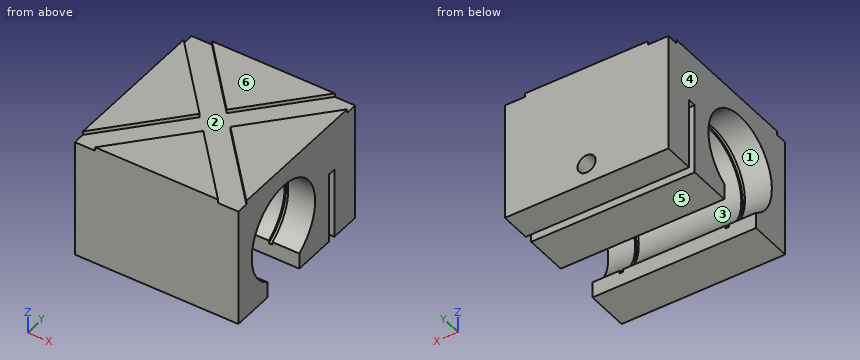
from build123d import *

# Parameters (mm, degrees)
SKETCH3_W               = 67
SKETCH3_H               = 50
BOSS_EXTRUDE1_DEPTH     = 70
CUT_EXTRUDE1_DEPTH      = 110.036691072
CUT_EXTRUDE1_DEPTH_BACK = 1.5
CUT_EXTRUDE3_DEPTH      = 110.036691072
SKETCH8_W               = 29
SKETCH8_H               = 3.3
CUT_EXTRUDE4_DEPTH      = 110.036691072
CUT_EXTRUDE5_REACH      = 111.037
SKETCH4_R               = 3.720223744
SKETCH9_R               = 20
CUT_EXTRUDE6_DEPTH      = 1.5
CUT_EXTRUDE7_START      = -1.5
SKETCH10_R              = 20
CUT_EXTRUDE7_DEPTH      = 1.5


with BuildPart() as part:
    # Sketch3 → Boss-Extrude1 (new body)
    with BuildSketch(Plane(origin=(0, 0, 0), x_dir=(1, 0, 0), z_dir=(0, 1, 0))):
        with Locations((33.5, 25)):
            Rectangle(SKETCH3_W, SKETCH3_H)
    extrude(amount=-BOSS_EXTRUDE1_DEPTH)

    # Sketch5 → Cut-Extrude1 (cut, two sides: drawn at the far end of the back side and taken through both)
    with BuildSketch(Plane.XY.offset(-CUT_EXTRUDE1_DEPTH_BACK)):
        Polygon((27.182851456, -35), (0, -65.2), (0, -70), (8.313843876, -70), (33.5, -42.018317645), (58.686156124, -70), (67, -70), (67, -65.2), (39.817148544, -35), (67, -4.8), (67, 0), (58.686156124, 0), (33.5, -27.981682355), (8.313843876, 0), (0, 0), (0, -4.8), align=None)
    extrude(amount=CUT_EXTRUDE1_DEPTH + CUT_EXTRUDE1_DEPTH_BACK, mode=Mode.SUBTRACT)

    # Sketch6 → Cut-Extrude3 (cut, through all)
    with BuildSketch(Plane(origin=(67, 0, 0), x_dir=(0, 0, -1), z_dir=(1, 0, 0))):
        with BuildLine():
            Line((43.454482672, -33.5), (50, -33.5))
            Line((50, -33.5), (50, -52.5))
            Line((50, -52.5), (43.454482672, -52.5))
            ThreePointArc((43.454482672, -52.5), (8, -43), (43.454482672, -33.5))
        make_face()
    extrude(amount=-CUT_EXTRUDE3_DEPTH, mode=Mode.SUBTRACT)

    # Sketch8 → Cut-Extrude4 (cut, through all)
    with BuildSketch(Plane(origin=(67, 0, 0), x_dir=(0, 0, -1), z_dir=(1, 0, 0))):
        with Locations((35.5, -14.15)):
            Rectangle(SKETCH8_W, SKETCH8_H)
    extrude(amount=-CUT_EXTRUDE4_DEPTH, mode=Mode.SUBTRACT)

    # Sketch4 → Cut-Extrude5 (cut, up to next)
    with BuildSketch(Plane(origin=(0, 0, 0), x_dir=(1, 0, 0), z_dir=(0, 1, 0)), mode=Mode.PRIVATE) as cut_extrude5_sk1:
        with Locations(Location((33.5, 41.7, 0), (0, 0, 270))):
            Circle(SKETCH4_R)
    cut_extrude5_tool1 = extrude(cut_extrude5_sk1.sketch, amount=-CUT_EXTRUDE5_REACH, mode=Mode.PRIVATE) & part.part
    add(cut_extrude5_tool1.solids().sort_by_distance((33.5, 0, -41.7))[0], mode=Mode.SUBTRACT)

    # Sketch9 → Cut-Extrude6 (cut)
    with BuildSketch(Plane(origin=(54.5, 0, 0), x_dir=(0, 0, -1), z_dir=(1, 0, 0))):
        with Locations((27, -43)):
            Circle(SKETCH9_R)
    extrude(amount=CUT_EXTRUDE6_DEPTH, mode=Mode.SUBTRACT)

    # Sketch10 → Cut-Extrude7 (cut)
    with BuildSketch(Plane(origin=(12.5, 0, 0), x_dir=(0, 0, -1), z_dir=(1, 0, 0)).offset(CUT_EXTRUDE7_START)):
        with Locations((27, -43)):
            Circle(SKETCH10_R)
    extrude(amount=CUT_EXTRUDE7_DEPTH, mode=Mode.SUBTRACT)


solid = part.part
The model under review builds one solid part; all positions refer to its coordinate system, in mm. Face numbers are marked on the shaded views. A direction names the side the tool comes from. Round coordinates to 2 decimals unless told otherwise and drop trailing zeros. Loops run counter-clockwise (first coordinate to the right, second up) from the corner with the lowest first, then second, coordinate; pieces in that order, holes last. Notation, with made-up numbers: M 26,70.5 L 36,70.5 A16 cw 36,82.5 Z; hole C 57.25,34 d7. An arc over 180 degrees is marked long. Answer as CSV lines item,"result".
1. We need section C-C (x = 32). Give the boundary of the cut face in (y, z), plus the area to 3 significant figures.
Outcome:
outline,"M -70,-50 L -52.5,-50 L -52.5,-43.45 A19 cw long -33.5,-43.45 L -33.5,-50 L -15.8,-50 L -15.8,-21 L -12.5,-21 L -12.5,-38.3 L 0,-38.3 L 0,0 L -26.32,0 L -26.32,-1.5 L -43.68,-1.5 L -43.68,0 L -70,0 Z; M -12.5,-50 L 0,-50 L 0,-45.1 L -12.5,-45.1 Z"
area,"2,070 mm2"
2. We need section A-A (z = -27). Give the boundary of the cut face in (x, y), plus the area to 3 significant figures.
Outcome:
outline,"M 0,-70 L 67,-70 L 67,-62 L 56,-62 L 56,-63 L 54.5,-63 L 54.5,-62 L 12.5,-62 L 12.5,-63 L 11,-63 L 11,-62 L 0,-62 Z; M 0,-24 L 11,-24 L 11,-23 L 12.5,-23 L 12.5,-24 L 54.5,-24 L 54.5,-23 L 56,-23 L 56,-24 L 67,-24 L 67,-15.8 L 0,-15.8 Z; M 0,-12.5 L 67,-12.5 L 67,0 L 0,0 Z"
area,"1,920 mm2"
3. Insertion check: pin 1 Ø6 at (x, y) = (22.5, -49.5) entering from +Z; pin 2 Ø1.7 at (x, y) = (43.5, -14) entering from -Z. Each pin has a flat end and moves straight along its axis. Give the tip position at first contact, or say it passes through.
Outcome:
pin 1,"stops at z = -1.5"
pin 2,"stops at z = -21"
4. We need section D-D (z = -13). Give the boundary of the cut face in (x, y).
Outcome:
outline,"M 0,-70 L 67,-70 L 67,-55.85 L 56,-55.85 L 56,-57.28 L 54.5,-57.28 L 54.5,-55.85 L 12.5,-55.85 L 12.5,-57.28 L 11,-57.28 L 11,-55.85 L 0,-55.85 Z; M 0,-30.15 L 11,-30.15 L 11,-28.72 L 12.5,-28.72 L 12.5,-30.15 L 54.5,-30.15 L 54.5,-28.72 L 56,-28.72 L 56,-30.15 L 67,-30.15 L 67,0 L 0,0 Z"
5. To check wall thickness, follow L1, parallel to Y at x = 54, z = -27; L2, parallel to Y at x = 54.95, z = -27; L3, parallel to X at y = -3.25, z = -41.7. State the ranges of each line that lie inside material, in increasing order. Write a range as [from, to].
Outcome:
L1,"y = [-70, -62], [-24, -15.8], [-12.5, 0]"
L2,"y = [-70, -63], [-23, -15.8], [-12.5, 0]"
L3,"x = [0, 29.78], [37.22, 67]"
6. For the marked faces 1 and 2, list the 3-axis set-ups (+Z, -Z, +X, -X, +Y, -Y) from which the entire face can be reached by the end or side of a thin tool; tool diameter is ignored.
Outcome:
face 1,"+X, -X"
face 2,"+Z"
7. Draft analysis for pull direction Z (two halves, no side actions). For the marked faces 3, 4, 5 and 6, state which applies: pulls with the +Z half, pulls with the -Z half, needs draft (parallel to the pull), parting line crosses it, or undercut.
Outcome:
face 3,"undercut"
face 4,"needs draft"
face 5,"pulls with the -Z half"
face 6,"pulls with the +Z half"
8. We need section B-B (y = -29). Give the boundary of the cut face in (x, z).
Outcome:
outline,"M 0,-50 L 67,-50 L 67,-39.85 L 56,-39.85 L 56,-41.28 L 54.5,-41.28 L 54.5,-39.85 L 12.5,-39.85 L 12.5,-41.28 L 11,-41.28 L 11,-39.85 L 0,-39.85 Z; M 0,-14.15 L 11,-14.15 L 11,-12.72 L 12.5,-12.72 L 12.5,-14.15 L 54.5,-14.15 L 54.5,-12.72 L 56,-12.72 L 56,-14.15 L 67,-14.15 L 67,0 L 45.22,0 L 45.22,-1.5 L 21.78,-1.5 L 21.78,0 L 0,0 Z"
